For this review, take the finished solid that the model builds, in its own axes (mm). A direction names the side the tool comes from. Give positions to 0.01 mm unless a question says otherwise; leave off trailing zeros. Loops run counter-clockwise (first coordinate to the right, second up) from the corner with the lowest first, then second, coordinate; pieces in that order, holes last. Notation, with made-up numbers: (-11, 33.5) - (2, 33.5) arc R27 cw to (2, 49.5) - close; hole circle Ø11 at (44.5, 37.25). An arc over 180 degrees is marked (long way). Put each result on its own line as item: value.
from build123d import *

# Parameters (mm, degrees)
SKIZZE1_W                       = 144
SKIZZE1_H                       = 57
AUFSATZ_LINEAR_AUSTRAGEN1_DEPTH = 25
SKIZZE2_W                       = 8
SKIZZE2_H                       = 8
SCHNITT_LINEAR_AUSTRAGEN4_DEPTH = 18
SKIZZE5_W                       = 140
SKIZZE5_H                       = 20
SKIZZE5_W_2                     = 125
SKIZZE5_H_2                     = 13
SCHNITT_LINEAR_AUSTRAGEN5_DEPTH = 23
SKIZZE6_R                       = 14
SKIZZE6_W                       = 31
SKIZZE6_H                       = 7.5
SCHNITT_LINEAR_AUSTRAGEN6_DEPTH = 2


with BuildPart() as part:
    # Skizze1 → Aufsatz-Linear austragen1 (new body)
    with BuildSketch(Plane.XY):
        with Locations((-30.959148289, 0.914772727)):
            Rectangle(SKIZZE1_W, SKIZZE1_H)
    extrude(amount=AUFSATZ_LINEAR_AUSTRAGEN1_DEPTH)

    # Skizze2 → Schnitt-Linear austragen4 (cut)
    with BuildSketch(Plane.XY.offset(25)):
        with Locations((37.040851711, 0.914772727)):
            Rectangle(SKIZZE2_W, SKIZZE2_H)
        with Locations((-98.959148289, 0.914772727)):
            Rectangle(SKIZZE2_W, SKIZZE2_H)
    extrude(amount=-SCHNITT_LINEAR_AUSTRAGEN4_DEPTH, mode=Mode.SUBTRACT)

    # Skizze5 → Schnitt-Linear austragen5 (cut)
    with BuildSketch(Plane(origin=(0, 0, 0), x_dir=(-1, 0, 0), z_dir=(0, 0, -1))):
        with Locations((30.959148289, 17.414772727)):
            Rectangle(SKIZZE5_W, SKIZZE5_H)
        with Locations((30.959148289, 0.914772727)):
            Rectangle(SKIZZE5_W_2, SKIZZE5_H_2)
        with Locations((30.959148289, -15.585227273)):
            Rectangle(SKIZZE5_W, SKIZZE5_H)
    extrude(amount=-SCHNITT_LINEAR_AUSTRAGEN5_DEPTH, mode=Mode.SUBTRACT)

    # Skizze6 → Schnitt-Linear austragen6 (cut)
    with BuildSketch(Plane(origin=(0, 29.414772727, 0), x_dir=(1, 0, 0), z_dir=(0, 1, 0))):
        with Locations((17.040851711, 0)):
            Circle(SKIZZE6_R)
        with Locations((-78.959148289, 0)):
            Circle(SKIZZE6_R)
        with Locations((-30.959148289, -3.75)):
            Rectangle(SKIZZE6_W, SKIZZE6_H)
    extrude(amount=-SCHNITT_LINEAR_AUSTRAGEN6_DEPTH, mode=Mode.SUBTRACT)


solid = part.part
1) Take a section at A-A on z = 19.5. State the section outline as (x, y) points.
Geometry check:
outline: (-102.96, -27.59) - (41.04, -27.59) - (41.04, -3.09) - (33.04, -3.09) - (33.04, 4.91) - (41.04, 4.91) - (41.04, 29.41) - (-102.96, 29.41) - (-102.96, 4.91) - (-94.96, 4.91) - (-94.96, -3.09) - (-102.96, -3.09) - close; hole (-100.96, -25.59) - (39.04, -25.59) - (39.04, -5.59) - (31.54, -5.59) - (31.54, 7.41) - (39.04, 7.41) - (39.04, 27.41) - (-100.96, 27.41) - (-100.96, 7.41) - (-93.46, 7.41) - (-93.46, -5.59) - (-100.96, -5.59) - close
2) Take a section at C-C on x = -52. State the section outline as (y, z) points, and give its area (3 significant figures).
Geometry check:
outline: (-27.59, 0) - (-25.59, 0) - (-25.59, 23) - (27.41, 23) - (27.41, 0) - (29.41, 0) - (29.41, 25) - (-27.59, 25) - close
area: 206 mm²
3) Wall thickness on line 1 (Y direction, x = -93.5, z = 17.75); line 2 (X direction, y = 20, z = 11.5); line 3 (X direction, y = -3.5, z = 8.25): over which ranges is each line inside the solid? List them lowest first.
Geometry check:
line 1: y = -27.59 to -25.59, -5.59 to 7.41, 27.41 to 29.41
line 2: x = -102.96 to -100.96, 39.04 to 41.04
line 3: x = -102.96 to -93.46, 31.54 to 41.04
4) Draft analysis for pull direction Y (two halves, no side actions). For faces 1 (the face through (-32, 29.415, 15)), 2 (the face through (33.041, 1, 16)), 3 (the face through (17, 28, 14)), state which applies: pulls with the +Y half, pulls with the -Y half, needs draft (parallel to the pull), parting line crosses it, or undercut.
Geometry check:
face 1: pulls with the +Y half
face 2: undercut
face 3: needs draft
5) Insertion check: pin 1 Ø4 at (y, z) = (1.5, 11.5) entering from +X; pin 2 Ø0.6 at (x, y) = (-25, 28.5) entering from -Z. Each pin has a flat end and moves straight along its axis. Give the tip position at first contact, or say it passes through.
Geometry check:
pin 1: stops at x = 33.04
pin 2: stops at z = 7.5
6) Take a section at B-B on y = 23. State the section outline as (x, z) points, and give its area (3 significant figures).
Geometry check:
outline: (-102.96, 0) - (-100.96, 0) - (-100.96, 23) - (39.04, 23) - (39.04, 0) - (41.04, 0) - (41.04, 25) - (-102.96, 25) - close
area: 380 mm²
7) For faces 4 (the face through (-94.959, 1, 16)), 5 (the face through (39.041, 17, 11)), 6 (the face through (37, 1, 7)), 7 (the face through (-31, -26, 0)), 8 (the face through (-79, 28, 14)), list the 3-axis set-ups (+Z, -Z, +X, -X, +Y, -Y) from which the entire face can be reached by the end or side of a thin tool; tool diameter is ignored.
Geometry check:
face 4: +Z, -X
face 5: -Z
face 6: +Z, +X
face 7: -Z, +X, -X, +Y, -Y
face 8: -Z, +Y
